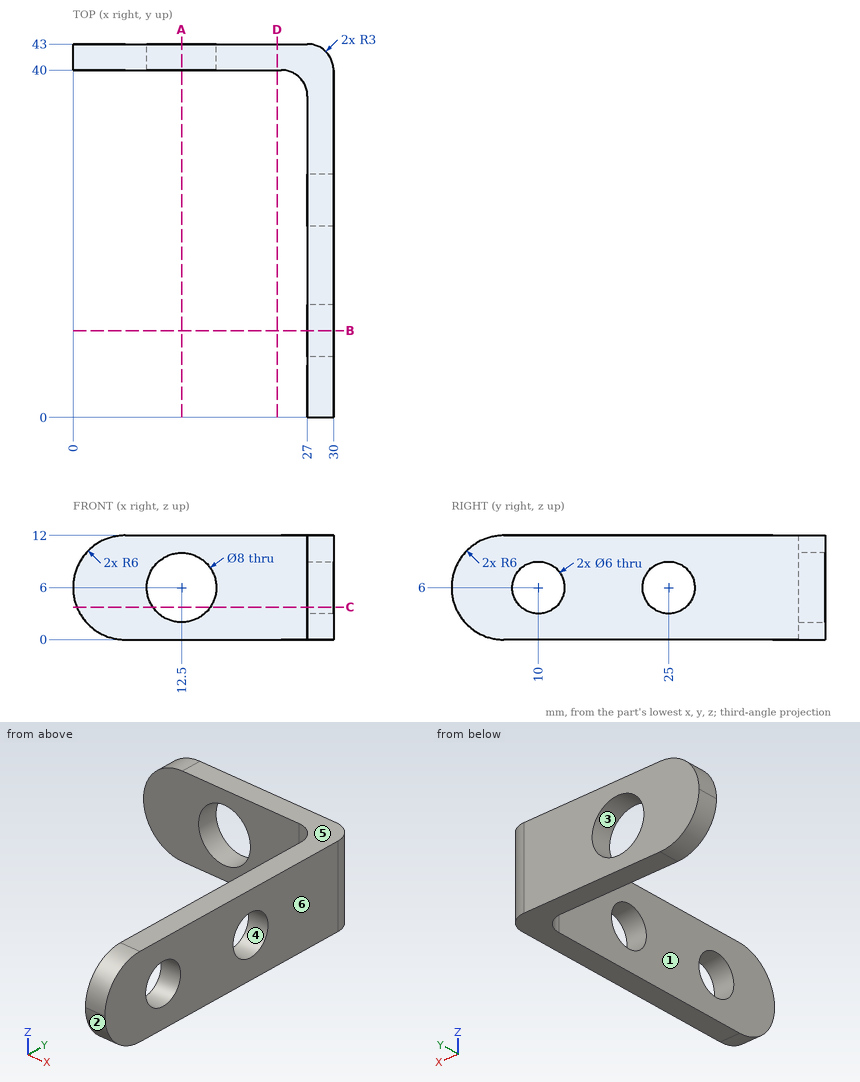
For this review, use the dimensioned drawing (mm, ordinates from the lowest corner) and the shaded views. A direction names the side the tool comes from. Round coordinates to 2 decimals unless told otherwise and drop trailing zeros. Loops run counter-clockwise (first coordinate to the right, second up) from the corner with the lowest first, then second, coordinate; pieces in that order, holes last. Notation, with made-up numbers: M -23,69 L 2,69 A10 ccw 2,87 Z; hole C 43.5,87.5 d5. An arc over 180 degrees is marked long. Answer as a JSON object with one key per item and string values.
(1) Clearance check with flat-ended pins moving along their axes: P1, Ø3.5, axis at y = 9.5, z = 3.5, coming from the -X side; P2, Ø5, axis at x = 21.5, z = 1.5, coming from the -Y side. State where each tip first meets the part, or that it passes through.
Resolved:
{"P1": "x = 27", "P2": "y = 40"}
(2) Draft analysis for pull direction Z (two halves, no side actions). For the marked faces 3, 4, 5 and 6, state which applies: released by +Z, released by -Z, zero draft, split by the parting line, or undercut.
Resolved:
{"face 3": "undercut", "face 4": "undercut", "face 5": "released by +Z", "face 6": "zero draft"}
(3) Tool access review of the marked faces 1 and 2: name each direction out of +Z, -Z, +X, -X, +Y, -Y from which nothing blocks a thin tool from reaching the whole face with its end or side.
Resolved:
{"face 1": "+Z, -Z, -X, -Y", "face 2": "-Z, +X, -X, -Y"}
(4) Take a section at D-D on x = 23.5. Give the boundary of the cut face in (y, z), and give its area (3 significant figures).
Resolved:
{"outline": "M 40,0 L 43,0 L 43,12 L 40,12 Z", "area": "36.0 mm²"}
(5) Take a section at B-B on y = 10. Give the boundary of the cut face in (x, z).
Resolved:
{"outline": "M 27,0 L 30,0 L 30,3 L 27,3 Z; M 27,9 L 30,9 L 30,12 L 27,12 Z"}
(6) Take a section at A-A on x = 12.5. Give the boundary of the cut face in (y, z).
Resolved:
{"outline": "M 40,0 L 43,0 L 43,2 L 40,2 Z; M 40,10 L 43,10 L 43,12 L 40,12 Z"}
(7) Take a section at C-C on z = 3.75. Give the boundary of the cut face in (x, y).
Resolved:
{"outline": "M 0.44,40 L 9.19,40 L 9.19,43 L 0.44,43 Z; M 15.81,40 L 24,40 A3 cw 27,37 L 27,26.98 L 30,26.98 L 30,40 A3 ccw 27,43 L 15.81,43 Z; M 27,0.44 L 30,0.44 L 30,8.02 L 27,8.02 Z; M 27,11.98 L 30,11.98 L 30,23.02 L 27,23.02 Z"}
(8) To check wall thickness, follow line 1 along X through (y, z) = (28, 10.25); line 2 along Y through (x, z) = (9.25, 2.75); line 3 along Y through (x, z) = (27.85, 6). State the ranges of each line that lie inside material, in increasing order.
Resolved:
{"line 1": "27 to 30", "line 2": "40 to 43", "line 3": "0 to 7, 13 to 22, 28 to 42.88"}
